Could you check a few things on this drawing? It's one solid part, dimensions in mm from its lowest x, y, z. A direction names the side the tool comes from. Coordinates: 2 decimals unless noted, no trailing zeros. Order: outer loops, then holes, each group sorted by start corner. A loop starts at its lowest first (then second) coordinate and runs counter-clockwise, first axis right, second up. Notation, with made-up numbers: (51, 13) -> (73, 13) arc R8 ccw to (73, 18) -> close; hole circle Ø11 at (78.5, 17.5). An arc over 180 degrees is marked (long way). Answer as CSV lines item,"result".
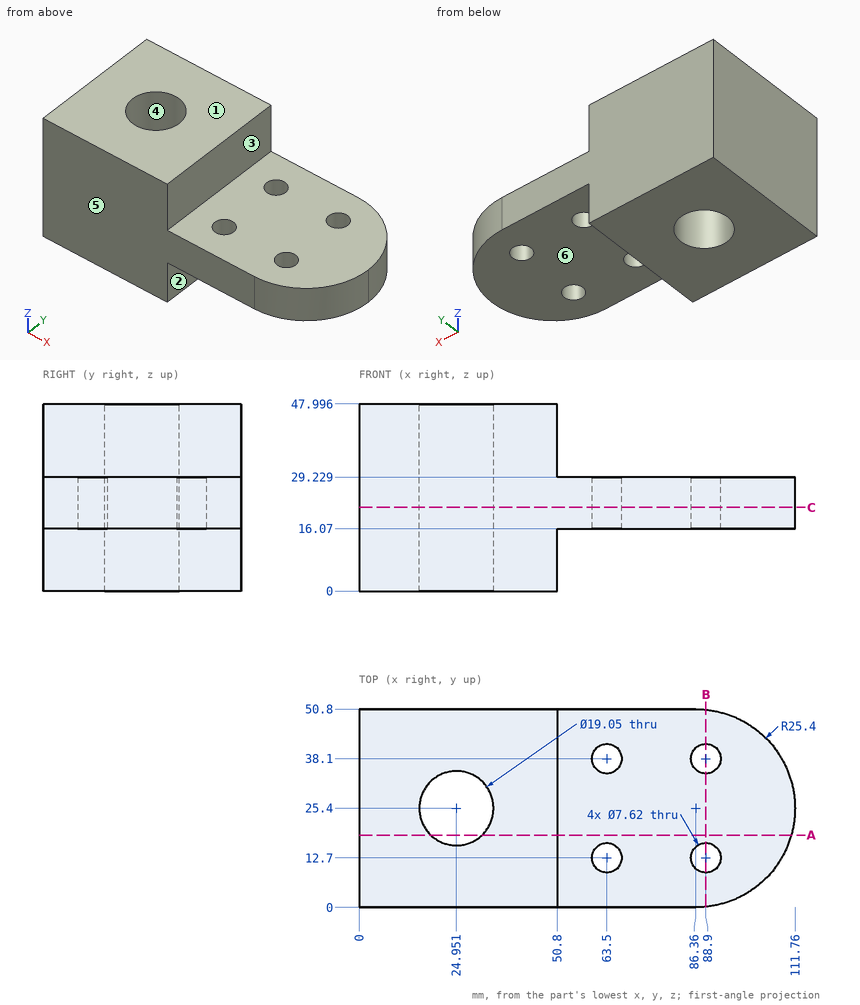
Q1. For P1, Ø10, axis at y = 24, z = 24.5, coming from the +X side; P2, Ø15, axis at x = 81, y = 22.5, coming from the -Z side; P3, Ø10, axis at y = 37, z = 7.5, coming from the +X side; P4, Ø3, axis at y = 32, z = 28.5, coming from the +X side, each with a flat end and sliding along its axis, tell me the tip position at first contact or that it passes through.
Solution:
P1,"x = 111.76"
P2,"z = 16.07"
P3,"x = 50.8"
P4,"x = 111.24"
Q2. If I drill on line 1 (Y direction, x = 63.5, z = 23.5); line 2 (X direction, y = 25, z = 29) (1 decimal); line 3 (X direction, y = 38, z = 26) (1 decimal), over which ranges is the centre line in solid material (lowest first)?
Solution:
line 1,"0 to 8.89, 16.51 to 34.29, 41.91 to 50.8"
line 2,"0 to 15.4, 34.5 to 111.8"
line 3,"0 to 59.7, 67.3 to 85.1, 92.7 to 108.4"
Q3. Imagine slicing it at C-C (z = 21.5). Give the number of separate pieces and of enclosed holes in the cut face, and give its area (3 significant figures).
Solution:
separate pieces,"1"
enclosed holes,"5"
area,"4,930 mm2"
Q4. Imagine slicing it at B-B (x = 88.9). List the corners of the cut face in (y, z) for me.
Solution:
outline,"(0.13, 16.07) -> (8.89, 16.07) -> (8.89, 29.23) -> (0.13, 29.23) -> close; (16.51, 16.07) -> (34.29, 16.07) -> (34.29, 29.23) -> (16.51, 29.23) -> close; (41.91, 16.07) -> (50.67, 16.07) -> (50.67, 29.23) -> (41.91, 29.23) -> close"
Q5. Imagine slicing it at A-A (y = 18.5). List the corners of the cut face in (x, z) for me (1 decimal), and give its area (3 significant figures).
Solution:
outline,"(0, 0) -> (18.4, 0) -> (18.4, 48) -> (0, 48) -> close; (31.5, 0) -> (50.8, 0) -> (50.8, 16.1) -> (110.8, 16.1) -> (110.8, 29.2) -> (50.8, 29.2) -> (50.8, 48) -> (31.5, 48) -> close"
area,"2,600 mm2"
Q6. Which directions (+Z, -Z, +X, -X, +Y, -Y) give clear straight access to the entire face, cutting with the end or side of a thin tool? Please do the marked faces 1, 2 and 3.
Solution:
face 1,"+Z, +X, -X, +Y, -Y"
face 2,"-Z, +X, +Y, -Y"
face 3,"+Z, +X, +Y, -Y"
Q7. We'd pull the mould along Y, two halves only. Please class the marked faces 4, 5 and 6: pulls with the +Y half, pulls with the -Y half, needs draft (parallel to the pull), parting line crosses it, or undercut.
Solution:
face 4,"undercut"
face 5,"pulls with the -Y half"
face 6,"needs draft"
